Here's how the part is built. I have some questions about the finished solid (model axes, mm). A direction names the side the tool comes from. Round coordinates to 2 decimals unless told otherwise and drop trailing zeros. Order: outer loops, then holes, each group sorted by start corner. A loop starts at its lowest first (then second) coordinate and runs counter-clockwise, first axis right, second up. Notation, with made-up numbers: (89, 49) -> (143, 49) arc R28 cw to (143, 84) -> close; hole circle Ø11 at (-35.75, 64.25). An arc over 180 degrees is marked (long way). One line per item, written item: value.
Autodesk Fusion 360 part; units mm, degrees
sketch "Boceto1" plane through (0, 0, 0) normal (0, 1, 0) x (1, 0, 0)
  circle A0 centre (100, -100) radius 100
extrude "Extruir1" add sketch "Boceto1" along normal blind 15
hole "Agujero1" at (100, 0, 100) direction (0, 1, 0) diameter 197 depth 197 tip angle 118
sketch "Boceto2" plane through (0, 0, 0) normal (0, 1, 0) x (1, 0, 0)
  circle A0 centre (100, -100) radius 100
  dimension "d6" = 200
extrude "Extruir2" cut sketch "Boceto1" along normal blind 0.003
extrude "Extruir3" add sketch "Boceto2" along normal blind 3
sketch "Boceto4" plane through (0, 3, 0) normal (0, 1, 0) x (-1, 0, 0)
  circle A0 centre (-100, 100) radius 98.5
  circle A1 centre (-100, 100) radius 15
  dimension "d11" = 30
extrude "Extruir4" add sketch "Boceto4" along normal blind 10 contours A1
shell "Vaciado1" thickness 12 removed faces 1 at (101.1126, 13, 95.1254)
extrude "Extruir5" cut 1 faces at (98.8219, 12, 99.3198) along direction (0, -1, 0) blind 5
hole "Agujero2" at (100, 9.0986, 97) direction (0, 0, -1) diameter 5 depth 3 tip angle 118
sketch "Boceto5" plane through (0, 7, 0) normal (0, 1, 0) x (-1, 0, 0)
  circle A0 centre (-100, 100) radius 3
  line L0 (-97.7639, 98) -> (-102.2361, 98)
extrude "Extruir6" add sketch "Boceto5" along normal blind 6 contours A0 L0 picked at (-100.6449, 97.9024)
sketch "Boceto6" plane through (0, 7, 0) normal (0, 1, 0) x (-1, 0, 0)
  line L0 (-102.2361, 98) -> (-97.7639, 98)
  arc A0 (-97.7639, 98) -> (-102.2361, 98) centre (-100, 100) ccw
  line L1 (-102.2361, 102) -> (-97.7639, 102)
extrude "Extruir7" add sketch "Boceto6" along normal blind 6 contours A0 L1
Q1. I want a section at B-B on x = 120. Write out the boundary of the cut face in (y, z).
Answers:
outline: (0, 2.02) -> (15, 2.02) -> (15, 3.55) -> (3, 3.55) -> (3, 196.45) -> (15, 196.45) -> (15, 197.98) -> (0, 197.98) -> close
Q2. I want a section at C-C on x = 88. Write out the boundary of the cut face in (y, z), then the cut area to 3 significant figures.
Answers:
outline: (0, 0.72) -> (15, 0.72) -> (15, 2.23) -> (3, 2.23) -> (3, 91) -> (13, 91) -> (13, 109) -> (3, 109) -> (3, 197.77) -> (15, 197.77) -> (15, 199.28) -> (0, 199.28) -> close
area: 812 mm2
Q3. I want a section at D-D on z = 107.5. Write out the boundary of the cut face in (x, y).
Answers:
outline: (0.28, 0) -> (199.72, 0) -> (199.72, 15) -> (198.21, 15) -> (198.21, 3) -> (112.99, 3) -> (112.99, 13) -> (87.01, 13) -> (87.01, 3) -> (1.79, 3) -> (1.79, 15) -> (0.28, 15) -> close
Q4. For P1, Ø2, axis at x = 160.5, y = 12, coming from the +Z side; P2, Ø5, axis at x = 177.5, z = 30, coming from the +Y side; P3, Ø6, axis at x = 136.5, y = 13, coming from the -Z side; P4, Ø3, axis at y = 4.5, z = 56.5, coming from the -X side, each with a flat end and sliding along its axis, tell me the tip position at first contact or that it passes through.
Answers:
P1: z = 180.37
P2: through
P3: z = 5.78
P4: x = 9.25
Q5. If we mould it in two halves opening along Y, with no side actions, what happens to faces 4 (the face through (100, 10, 102)), 5 (the face through (100, 13, 97)), 6 (the face through (100.37, 8.87, 92.76))? For each: pulls with the +Y half, pulls with the -Y half, needs draft (parallel to the pull), parting line crosses it, or undercut.
Answers:
face 4: needs draft
face 5: pulls with the +Y half
face 6: undercut
Q6. I want a section at A-A on z = 185.5. Write out the boundary of the cut face in (x, y).
Answers:
outline: (48.14, 0) -> (151.86, 0) -> (151.86, 15) -> (148.91, 15) -> (148.91, 3) -> (51.09, 3) -> (51.09, 15) -> (48.14, 15) -> close
Q7. Which directions (+Z, -Z, +X, -X, +Y, -Y) give clear straight access to the entire face, cutting with the end or side of a thin tool? Please do faces 1 (the face through (97.52, 9.42, 95.48)), 2 (the face through (99, 0, 99)), 3 (the face through (121, 3, 99)).
Answers:
face 1: none
face 2: +Z, -Z, +X, -X, -Y
face 3: +Y
Q8. I need wall thicknesses on line 1 along Y through (x, z) = (100, 95.55); line 2 along Z through (x, y) = (100, 11.5); line 3 along Y through (x, z) = (185.5, 56). Which ranges of each line are inside material? Lowest first, please.
Answers:
line 1: 0 to 6.6, 11.6 to 13
line 2: 0 to 1.5, 85 to 93.94, 97 to 98, 102 to 115, 198.5 to 200
line 3: 0 to 3
